from build123d import *

# Parameters (mm, degrees)
SKETCH1_R           = 9.5
BOSS_EXTRUDE1_DEPTH = 16
SKETCH1_3_R         = 10.75
SKETCH1_3_R_2       = 9.5
BOSS_EXTRUDE2_DEPTH = 11.5
SKETCH2_R           = 2.25
CUT_EXTRUDE1_DEPTH  = 23.070908454
SKETCH3_R           = 1.35
CUT_EXTRUDE2_DEPTH  = 23.070908454
CUT_EXTRUDE7_DEPTH  = 9
CUT_EXTRUDE8_DEPTH  = 6.1
BOSS_EXTRUDE5_START = 2
SKETCH8_R           = 2.25
BOSS_EXTRUDE5_DEPTH = 2
BOSS_EXTRUDE6_START = 2
SKETCH9_R           = 10.75
BOSS_EXTRUDE6_DEPTH = 2


with BuildPart() as part:
    # Sketch1 → Boss-Extrude1 (new body)
    with BuildSketch(Plane.XY):
        Circle(SKETCH1_R)
    extrude(amount=-BOSS_EXTRUDE1_DEPTH)

    # Sketch1_3 → Boss-Extrude2 (add)
    with BuildSketch(Plane.XY):
        Circle(SKETCH1_3_R)
        Circle(SKETCH1_3_R_2, mode=Mode.SUBTRACT)
    extrude(amount=-BOSS_EXTRUDE2_DEPTH)

    # Sketch2 → Cut-Extrude1 (cut, through all)
    with BuildSketch(Plane.XY):
        Circle(SKETCH2_R)
    extrude(amount=-CUT_EXTRUDE1_DEPTH, mode=Mode.SUBTRACT)

    # Sketch3 → Cut-Extrude2 (cut, through all)
    with BuildSketch(Plane(origin=(0, 0, -16), x_dir=(-1, 0, 0), z_dir=(0, 0, -1))):
        with Locations((0, 6.5)):
            Circle(SKETCH3_R)
        with Locations((-6.5, 0)):
            Circle(SKETCH3_R)
        with Locations((6.5, 0)):
            Circle(SKETCH3_R)
        with Locations((0, -6.5)):
            Circle(SKETCH3_R)
    extrude(amount=-CUT_EXTRUDE2_DEPTH, mode=Mode.SUBTRACT)

    # Sketch5 → Cut-Extrude7 (cut)
    with BuildSketch(Plane.XY):
        Polygon((1.241303079, 4.35), (2.482606158, 6.5), (1.241303079, 8.65), (-1.241303079, 8.65), (-2.482606158, 6.5), (-1.241303079, 4.35), align=None)
        Polygon((-5.258696921, -2.15), (-4.017393842, 0), (-5.258696921, 2.15), (-7.741303079, 2.15), (-8.982606158, 0), (-7.741303079, -2.15), align=None)
        Polygon((1.241303079, -8.65), (2.482606158, -6.5), (1.241303079, -4.35), (-1.241303079, -4.35), (-2.482606158, -6.5), (-1.241303079, -8.65), align=None)
        Polygon((7.741303079, -2.15), (8.982606158, 0), (7.741303079, 2.15), (5.258696921, 2.15), (4.017393842, 0), (5.258696921, -2.15), align=None)
    extrude(amount=-CUT_EXTRUDE7_DEPTH, mode=Mode.SUBTRACT)

    # Sketch6 → Cut-Extrude8 (cut)
    with BuildSketch(Plane.XY):
        Polygon((3.492969129, -6.05), (6.985938257, 0), (3.492969129, 6.05), (-3.492969129, 6.05), (-6.985938257, 0), (-3.492969129, -6.05), align=None)
    extrude(amount=-CUT_EXTRUDE8_DEPTH, mode=Mode.SUBTRACT)

    # Sketch8 → Boss-Extrude5 (add)
    with BuildSketch(Plane.XY.offset(-6.1).offset(BOSS_EXTRUDE5_START)):
        Polygon((-1.241303079, 4.35), (-2.222798536, 6.05), (-3.492969129, 6.05), (-5.744635178, 2.15), (-5.258696921, 2.15), (-4.017393842, 0), (-5.258696921, -2.15), (-5.744635178, -2.15), (-3.492969129, -6.05), (-2.222798536, -6.05), (-1.241303079, -4.35), (1.241303079, -4.35), (2.222798536, -6.05), (3.492969129, -6.05), (5.744635178, -2.15), (5.258696921, -2.15), (4.017393842, 0), (5.258696921, 2.15), (5.744635178, 2.15), (3.492969129, 6.05), (2.222798536, 6.05), (1.241303079, 4.35), align=None)
        Circle(SKETCH8_R, mode=Mode.SUBTRACT)
    extrude(amount=-BOSS_EXTRUDE5_DEPTH)

    # Sketch9 → Boss-Extrude6 (add)
    with BuildSketch(Plane.XY.offset(BOSS_EXTRUDE6_START)):
        Circle(SKETCH9_R)
        Polygon((-3.492969129, 6.05), (-5.744635178, 2.15), (-7.741303079, 2.15), (-8.982606158, 0), (-7.741303079, -2.15), (-5.744635178, -2.15), (-3.492969129, -6.05), (-2.222798536, -6.05), (-2.482606158, -6.5), (-1.241303079, -8.65), (1.241303079, -8.65), (2.482606158, -6.5), (2.222798536, -6.05), (3.492969129, -6.05), (5.744635178, -2.15), (7.741303079, -2.15), (8.982606158, 0), (7.741303079, 2.15), (5.744635178, 2.15), (3.492969129, 6.05), (2.222798536, 6.05), (2.482606158, 6.5), (1.241303079, 8.65), (-1.241303079, 8.65), (-2.482606158, 6.5), (-2.222798536, 6.05), align=None, mode=Mode.SUBTRACT)
    extrude(amount=-BOSS_EXTRUDE6_DEPTH)


solid = part.part
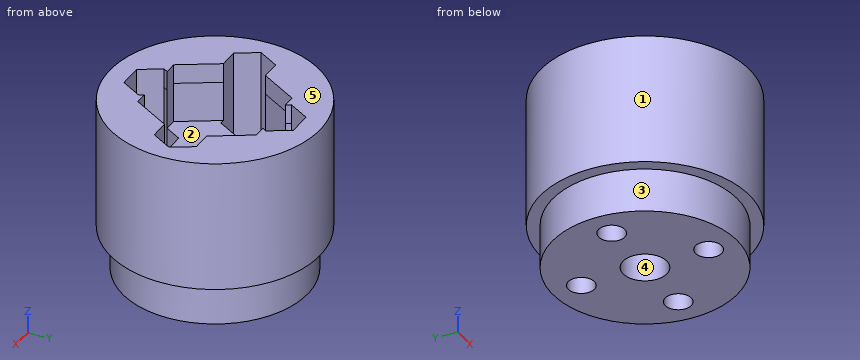
Verification items for the finished model (mm, model axes). Face numbers are marked on the shaded views. A direction names the side the tool comes from. Round coordinates to 2 decimals unless told otherwise and drop trailing zeros. Order: outer loops, then holes, each group sorted by start corner. A loop starts at its lowest first (then second) coordinate and runs counter-clockwise, first axis right, second up.
1. Access from +Z, -Z, +X, -X, +Y, -Y to the whole of each face (thin tool, end or side, straight path). Record for the marked faces 1 and 2.
Final values:
face 1: +Z, -Z
face 2: +Z
2. Section check B-B on z = -2.5. Record the cut outline in (x, y), then the cut area to 3 significant figures.
Final values:
outline: circle Ø21.5 at (0, 0); hole (-8.98, 0) - (-7.74, -2.15) - (-5.74, -2.15) - (-3.49, -6.05) - (-2.22, -6.05) - (-2.48, -6.5) - (-1.24, -8.65) - (1.24, -8.65) - (2.48, -6.5) - (2.22, -6.05) - (3.49, -6.05) - (5.74, -2.15) - (7.74, -2.15) - (8.98, 0) - (7.74, 2.15) - (5.74, 2.15) - (3.49, 6.05) - (2.22, 6.05) - (2.48, 6.5) - (1.24, 8.65) - (-1.24, 8.65) - (-2.48, 6.5) - (-2.22, 6.05) - (-3.49, 6.05) - (-5.74, 2.15) - (-7.74, 2.15) - close
area: 199 mm2
3. Section check D-D on y = 5.75. Record the cut outline in (x, z).
Final values:
outline: (-9.08, -11.5) - (-7.56, -11.5) - (-7.56, -16) - (-1.12, -16) - (-1.12, -9) - (-2.05, -9) - (-2.05, -4.1) - (-3.67, -4.1) - (-3.67, 2) - (-9.08, 2) - close; (1.12, -16) - (7.56, -16) - (7.56, -11.5) - (9.08, -11.5) - (9.08, 2) - (3.67, 2) - (3.67, -4.1) - (2.05, -4.1) - (2.05, -9) - (1.12, -9) - close
4. Thickness scan on L1, parallel to Y at x = 0, z = -8.5; L2, parallel to Y at x = 0, z = -12; L3, parallel to Z at x = 3.25, y = -3.5. Record the ranges inside material, lowest first.
Final values:
L1: y = -10.75 to -8.65, -4.35 to -2.25, 2.25 to 4.35, 8.65 to 10.75
L2: y = -9.5 to -7.85, -5.15 to -2.25, 2.25 to 5.15, 7.85 to 9.5
L3: z = -16 to -4.1
5. Go/stop test with flat-tipped pins: P1, Ø8, axis at y = 2.5, z = -12.5, coming from the -X side; P2, Ø2, axis at y = -3, z = -0.5, coming from the +X side; P3, Ø3.5, axis at x = 2.5, y = -2.5, coming from the +Z side; P4, Ø1, axis at x = -3, z = -0.5, coming from the +Y side. Record where each tip stops, or that it passes through.
Final values:
P1: stops at x = -10.75
P2: stops at x = 10.56
P3: stops at z = -4.1
P4: stops at y = 10.46
6. Release check for a two-part mould opening along Y. For the marked faces 3, 4 and 5 record: +Y half, -Y half, draft (parallel to the pull), parting line (faces both ways), or undercut.
Final values:
face 3: parting line
face 4: undercut
face 5: draft
7. Section check C-C on z = -8. Record the cut outline in (x, y), then the cut area to 3 significant figures.
Final values:
outline: circle Ø21.5 at (0, 0); hole (-8.98, 0) - (-7.74, -2.15) - (-5.26, -2.15) - (-4.02, 0) - (-5.26, 2.15) - (-7.74, 2.15) - close; hole (-2.48, -6.5) - (-1.24, -8.65) - (1.24, -8.65) - (2.48, -6.5) - (1.24, -4.35) - (-1.24, -4.35) - close; hole (-2.48, 6.5) - (-1.24, 4.35) - (1.24, 4.35) - (2.48, 6.5) - (1.24, 8.65) - (-1.24, 8.65) - close; hole circle Ø4.5 at (0, 0); hole (4.02, 0) - (5.26, -2.15) - (7.74, -2.15) - (8.98, 0) - (7.74, 2.15) - (5.26, 2.15) - close
area: 283 mm2
8. Section check A-A on x = 0. Record the cut outline in (y, z).
Final values:
outline: (-10.75, -11.5) - (-9.5, -11.5) - (-9.5, -16) - (-7.85, -16) - (-7.85, -9) - (-8.65, -9) - (-8.65, 2) - (-10.75, 2) - close; (-5.15, -16) - (-2.25, -16) - (-2.25, -4.1) - (-4.35, -4.1) - (-4.35, -9) - (-5.15, -9) - close; (2.25, -16) - (5.15, -16) - (5.15, -9) - (4.35, -9) - (4.35, -4.1) - (2.25, -4.1) - close; (7.85, -16) - (9.5, -16) - (9.5, -11.5) - (10.75, -11.5) - (10.75, 2) - (8.65, 2) - (8.65, -9) - (7.85, -9) - close
